from build123d import *

# Parameters (mm, degrees)
F0_W      = 530
F0_H      = 130
F1_DEPTH  = 30
F2_R      = 3
F3_DEPTH  = 12
F4_R      = 3
F5_DEPTH  = 11
F6_R      = 3
F7_DEPTH  = 12
F8_R      = 3
F9_DEPTH  = 10
F10_R     = 3
F11_DEPTH = 12


with BuildPart() as f1:
    # F0 (on Right) → F1 (new body)
    with BuildSketch(Plane.YZ):
        with Locations((265, 65)):
            Rectangle(F0_W, F0_H)
    extrude(amount=F1_DEPTH)

    # F2 (on face) → F3 (cut)
    with BuildSketch(Plane(origin=(0, 0, 0), x_dir=(1, 0, 0), z_dir=(0, 0, -1))):
        with Locations((15, -130)):
            Circle(F2_R)
    extrude(amount=-F3_DEPTH, mode=Mode.SUBTRACT)

    # F4 (on face) → F5 (cut)
    with BuildSketch(Plane(origin=(0, 0, 0), x_dir=(1, 0, 0), z_dir=(0, 0, -1))):
        with Locations((15, -400)):
            Circle(F4_R)
    extrude(amount=-F5_DEPTH, mode=Mode.SUBTRACT)

    # F6 (on face) → F7 (cut)
    with BuildSketch(Plane.XY.offset(130)):
        with Locations((15, 130)):
            Circle(F6_R)
        with Locations((15, 400)):
            Circle(F6_R)
    extrude(amount=-F7_DEPTH, mode=Mode.SUBTRACT)

    # F8 (on face) → F9 (cut)
    with BuildSketch(Plane.YZ.offset(30)):
        with Locations((400, 15)):
            Circle(F8_R)
        with Locations((130, 15)):
            Circle(F8_R)
    extrude(amount=-F9_DEPTH, mode=Mode.SUBTRACT)

    # F10 (on face) → F11 (cut)
    with BuildSketch(Plane.YZ.offset(30)):
        with Locations((15, 65)):
            Circle(F10_R)
    extrude(amount=-F11_DEPTH, mode=Mode.SUBTRACT)


solid = f1.part
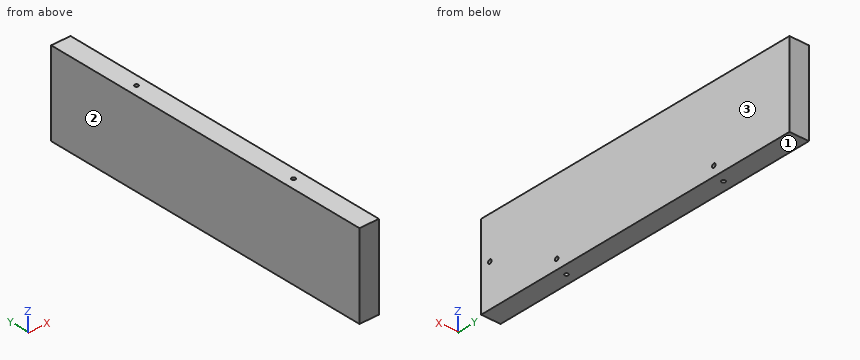
Verification items for the finished model (mm, model axes). Face numbers are marked on the shaded views. Give positions to 0.01 mm unless a question says otherwise; leave off trailing zeros. Answer as CSV lines item,"result". Start each with the question number.
1. Draft check along X on the marked faces 1, 2 and 3. Enter one of: pulls with the +X half, pulls with the -X half, needs draft (parallel to the pull), parting line crosses it, or undercut.
2. Thickness scan on line 1 (Y direction, x = 15, z = 8.5); line 2 (Z direction, x = 26, y = 130); line 3 (Z direction, x = 20.5, y = 15). Record the ranges inside material, lowest first.
3. Depth check by flat-ended pin: pin 1 (5.5 mm diameter, centred on x = 15, y = 130, fed in from -Z); pin 2 (3.5 mm diameter, centred on x = 15, y = 400, fed in from +Z); pin 3 (1.8 mm diameter, centred on y = 399.5, z = 15.5, fed in from +X). Enter the tip coordinate at first touch or a pass-through.
Derived:
1,face 1,"needs draft"
1,face 2,"pulls with the -X half"
1,face 3,"pulls with the +X half"
2,line 1,"0 to 127, 133 to 397, 403 to 530"
2,line 2,"0 to 12, 18 to 130"
2,line 3,"0 to 62, 68 to 130"
3,pin 1,"z = 12"
3,pin 2,"z = 118"
3,pin 3,"x = 20"
